Drawing for the job (mm, zero at the part's lowest x, y, z). A direction names the side the tool comes from. Round coordinates to 2 decimals unless told otherwise and drop trailing zeros. Write each loop counter-clockwise with the first axis right and the second up, starting at its lowest first coordinate (ties: lowest second). Pieces come first, ordered by that corner, then holes. Notation, with made-up numbers: (4, 50) - (10, 50) arc R19 ccw to (10, 54) - close; hole circle Ø4 at (-31.75, 45.25). An arc over 180 degrees is marked (long way). One line per question, with ' | ' between items.
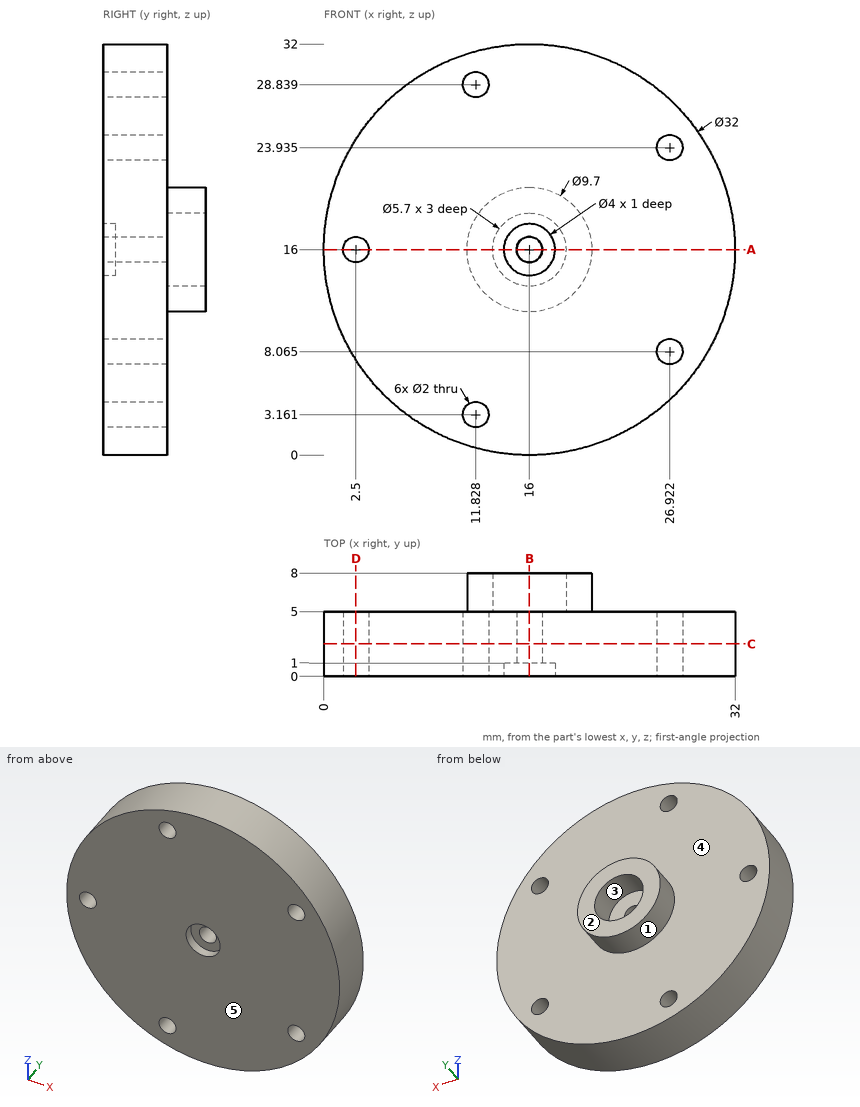
Q1. Saw through at B-B, the plane x = 16. List the corners of the cut face in (y, z), then the cut area to 3 significant figures.
Found:
outline: (0, 0) - (5, 0) - (5, 11.15) - (8, 11.15) - (8, 13.15) - (5, 13.15) - (5, 15) - (1, 15) - (1, 14) - (0, 14) - close; (0, 18) - (1, 18) - (1, 17) - (5, 17) - (5, 18.85) - (8, 18.85) - (8, 20.85) - (5, 20.85) - (5, 32) - (0, 32) - close | area: 160 mm^2
Q2. Pull direction Z, two halves, no side cores. Call the marked faces 1, 2 and 3: +Z half, -Z half, draft (parallel to the pull), parting line (faces both ways), or undercut.
Found:
face 1: parting line | face 2: draft | face 3: undercut
Q3. Drop flat-ended pins along their axis: pin 1 (3 mm diameter, centred on x = 26.92, z = 23.94, fed in from -Y); pin 2 (4 mm diameter, centred on y = 2, z = 19.5, fed in from +X); pin 3 (1 mm diameter, centred on x = 20, y = 2, fed in from +Z); pin 4 (1.7 mm diameter, centred on x = 17, z = 15.5, fed in from +Y). Give the stop position or say it passes through.
Found:
pin 1: y = 0 | pin 2: x = 31.93 | pin 3: z = 31.61 | pin 4: y = 5
Q4. Saw through at C-C, the plane y = 2.5. List the corners of the cut face in (x, z) (1 decimal).
Found:
outline: circle Ø32 at (16, 16); hole circle Ø2 at (2.5, 16); hole circle Ø2 at (11.8, 3.2); hole circle Ø2 at (11.8, 28.8); hole circle Ø2 at (16, 16); hole circle Ø2 at (26.9, 8.1); hole circle Ø2 at (26.9, 23.9)
Q5. Drill centre lines: L1, parallel to X at y = 3.5, z = 16; L2, parallel to Y at x = 7, z = 25.5; L3, parallel to X at y = 1.5, z = 4 (1 decimal). Where is each one in solid material? Low to high. Write a range as from..to.
Found:
L1: 0..1.5, 3.5..15, 17..32 | L2: 0..5 | L3: 5.4..11.3, 12.4..26.6
Q6. Saw through at D-D, the plane x = 2.5. List the corners of the cut face in (y, z), then the cut area to 3 significant figures.
Found:
outline: (0, 7.41) - (5, 7.41) - (5, 15) - (0, 15) - close; (0, 17) - (5, 17) - (5, 24.59) - (0, 24.59) - close | area: 75.9 mm^2
Q7. Which spindle directions (+Z, -Z, +X, -X, +Y, -Y) get a long thin tool onto all of the face, cutting with end or side? Do the marked faces 4 and 5. Say none if no direction does.
Found:
face 4: +Y | face 5: +Z, -Z, +X, -X, -Y
Q8. Saw through at A-A, the plane z = 16. List the corners of the cut face in (x, y), then the cut area to 3 significant figures.
Found:
outline: (0, 0) - (1.5, 0) - (1.5, 5) - (0, 5) - close; (3.5, 0) - (14, 0) - (14, 1) - (15, 1) - (15, 5) - (13.15, 5) - (13.15, 8) - (11.15, 8) - (11.15, 5) - (3.5, 5) - close; (17, 1) - (18, 1) - (18, 0) - (32, 0) - (32, 5) - (20.85, 5) - (20.85, 8) - (18.85, 8) - (18.85, 5) - (17, 5) - close | area: 150 mm^2
